Input: dimensioned drawing with shaded views. Units: mm. Origin: part minimum x, y, z. A direction names the side the tool comes from. Round coordinates to 2 decimals unless told otherwise and drop trailing zeros. Loops run counter-clockwise (first coordinate to the right, second up) from the corner with the lowest first, then second, coordinate; pieces in that order, holes last. Notation, with made-up numbers: (21.5, 75) - (63.5, 75) arc R27 cw to (63.5, 97) - close; hole circle Ø11 at (14, -29). An arc over 180 degrees is marked (long way). One line per question, with ' | ' between items.
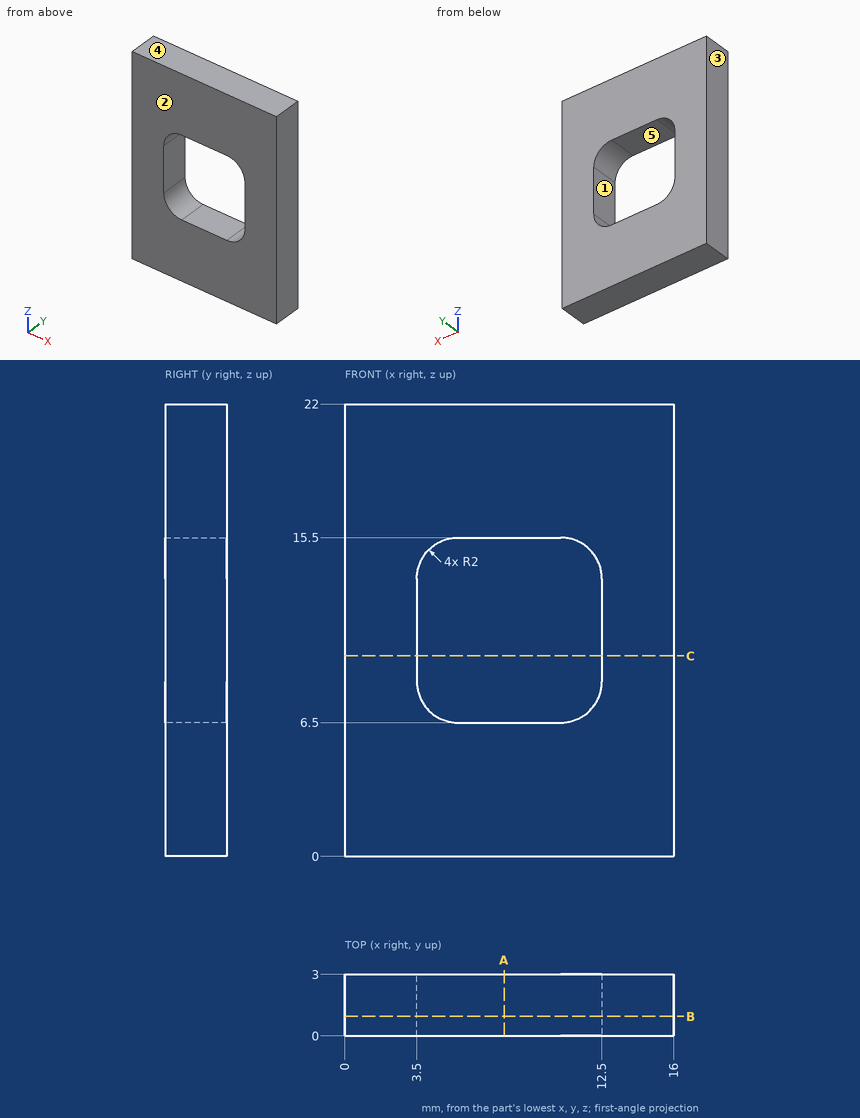
1. Mould query, pull axis Z, two halves, no side actions, for the marked faces 3, 4 and 5. Classes: released by +Z, released by -Z, zero draft, split by the parting line, or undercut.
Worked out:
face 3: zero draft | face 4: released by +Z | face 5: undercut
2. Material intervals for probe 1 along X at (y, z) = (1.45, 9.5); probe 2 along Z at (x, y) = (7.25, 2.2); probe 3 along Z at (x, y) = (11.5, 2.1), sorted ascending.
Worked out:
probe 1: x = 0 to 3.5, 12.5 to 16 | probe 2: z = 0 to 6.5, 15.5 to 22 | probe 3: z = 0 to 6.77, 15.23 to 22
3. Access query for the marked faces 1 and 2. Directions: +Z, -Z, +X, -X, +Y, -Y. A direction counts if a zero-diameter tool reaches every point of the face in a straight line with its end or side. Return the directions, or none.
Worked out:
face 1: +Y, -Y | face 2: +Z, -Z, +X, -X, -Y
4. Section query C-C, the plane z = 9.75. Return loops of the section in (x, y).
Worked out:
outline: (0, 0) - (3.5, 0) - (3.5, 3) - (0, 3) - close; (12.5, 0) - (16, 0) - (16, 3) - (12.5, 3) - close
5. Section query A-A, the plane x = 7.75. Return loops of the section in (y, z).
Worked out:
outline: (0, 0) - (3, 0) - (3, 6.5) - (0, 6.5) - close; (0, 15.5) - (3, 15.5) - (3, 22) - (0, 22) - close
6. Section query B-B, the plane y = 0.95. Return loops of the section in (x, z).
Worked out:
outline: (0, 0) - (16, 0) - (16, 22) - (0, 22) - close; hole (3.5, 8.5) arc R2 ccw to (5.5, 6.5) - (10.5, 6.5) arc R2 ccw to (12.5, 8.5) - (12.5, 13.5) arc R2 ccw to (10.5, 15.5) - (5.5, 15.5) arc R2 ccw to (3.5, 13.5) - close
